Geometry: final body of the model. Coordinates: model frame, mm. A direction names the side the tool comes from. Round coordinates to 2 decimals unless told otherwise and drop trailing zeros. Write each loop counter-clockwise with the first axis right and the second up, starting at its lowest first coordinate (ties: lowest second). Pieces come first, ordered by that corner, then holes. Notation, with made-up numbers: (-10, 79.25) - (18, 79.25) arc R11 ccw to (18, 96.25) - close; hole circle Ø4 at (-29, 52.25). An arc over 180 degrees is marked (long way). Write each question's results on one line, items separated by ' | '.
from build123d import *

# Parameters (mm, degrees)
F2_R     = 5
F3_DEPTH = 25.001
F4_R     = 3
F5_DEPTH = 25.001
F6_R     = 4
F6_R_2   = 3
F7_DEPTH = 25
F7_TAPER = 1.2


with BuildPart() as f1:
    # F0 (on Front) → F1 (revolve)
    with BuildSketch(Plane.XZ):
        Polygon((20, 0), (0, 0), (0, -25), (15, -25), (15, -1), (17.1, -1), (17.1, -12), (20, -12), align=None)
    revolve(axis=Axis((0, 0, -20.7611778751), (0, 0, -1)))

    # F2 (on Top) → F3 (cut, through all)
    with BuildSketch(Plane.XY):
        Circle(F2_R)
    extrude(amount=-F3_DEPTH, mode=Mode.SUBTRACT)

    # F4 (on face) → F5 (cut, through all)
    with BuildSketch(Plane.XY):
        with Locations((-10, 0)):
            Circle(F4_R)
    extrude(amount=-F5_DEPTH, mode=Mode.SUBTRACT)

    # F6 (on face) → F7 (join)
    with BuildSketch(Plane.XY):
        with Locations((-10, 0)):
            Circle(F6_R)
        with Locations((-10, 0)):
            Circle(F6_R_2, mode=Mode.SUBTRACT)
    extrude(amount=F7_DEPTH, taper=F7_TAPER)


solid = f1.part
Q1. Ray query, line 1 along Y through (x, z) = (0, -9.5); line 2 along X through (y, z) = (4.5, -4); line 3 along X through (y, z) = (9, -7.5). Return the intervals inside material, ascending.
Answer block:
line 1: -20 to -17.1, -15 to -5, 5 to 15, 17.1 to 20 | line 2: -19.49 to -16.5, -14.31 to -2.18, 2.18 to 14.31, 16.5 to 19.49 | line 3: -17.86 to -14.54, -12 to 12, 14.54 to 17.86
Q2. Section query C-C, the plane y = 0. Give the number of separate pieces and of enclosed holes in the cut face, plus the area to 3 significant figures.
Answer block:
separate pieces: 3 | enclosed holes: 0 | area: 448 mm2
Q3. Section query D-D, the plane x = 7. Return loops of the section in (y, z) (1 decimal).
Answer block:
outline: (-18.7, -12) - (-15.6, -12) - (-15.6, -1) - (-13.3, -1) - (-13.3, -25) - (13.3, -25) - (13.3, -1) - (15.6, -1) - (15.6, -12) - (18.7, -12) - (18.7, 0) - (-18.7, 0) - close
Q4. Pin query (flat end, axial travel): pin 1 (8 mm diameter, centred on x = -3.5, z = -13, fed in from +Y); pin 2 (20 mm diameter, centred on x = 5.5, y = 2, fed in from +Z); pin 3 (6 mm diameter, centred on y = -4, z = -20, fed in from -X). Return the tip coordinate at first contact, or that it passes through.
Answer block:
pin 1: y = 20 | pin 2: z = 0 | pin 3: x = -14.97
Q5. Section query A-A, the plane x = 0. Return loops of the section in (y, z), plus the area to 3 significant figures.
Answer block:
outline: (-20, -12) - (-17.1, -12) - (-17.1, -1) - (-15, -1) - (-15, -25) - (-5, -25) - (-5, 0) - (-20, 0) - close; (5, -25) - (15, -25) - (15, -1) - (17.1, -1) - (17.1, -12) - (20, -12) - (20, 0) - (5, 0) - close | area: 574 mm2
Q6. Mould query, pull axis X, two halves, no side actions, for faces 1 (the cylindrical face through (-1.08, -4.88, -12.32)), 2 (the flat face through (-15, -9, -12)), 3 (the cylindrical face through (-4.336, 19.524, -5.916)). Classes: pulls with the +X half, pulls with the -X half, needs draft (parallel to the pull), parting line crosses it, or undercut.
Answer block:
face 1: undercut | face 2: needs draft | face 3: parting line crosses it
Q7. Section query B-B, the plane z = -15. Return loops of the section in (x, y), plus the area to 3 significant figures.
Answer block:
outline: circle Ø30 at (0, 0); hole circle Ø6 at (-10, 0); hole circle Ø10 at (0, 0) | area: 600 mm2
Q8. Access query for faces 4 (the flat face through (4, -4, -25)), 5 (the conical face through (-6.43, 1.13, 12.1)), 6 (the cylindrical face through (-14.985, -0.66, -12.832)). Directions: +Z, -Z, +X, -X, +Y, -Y. A direction counts if a zero-diameter tool reaches every point of the face in a straight line with its end or side. Return the directions, or none.
Answer block:
face 4: -Z, +X, -X, +Y, -Y | face 5: +Z | face 6: -Z
